```python
from build123d import *

# Parameters (mm, degrees)
EXTRUDE_2_DEPTH = 350
FILLET_1_R      = 1.5


with BuildPart() as part:
    # 草图1 → 凸台-拉伸2 (new body)
    with BuildSketch(Plane.XY):
        Polygon((-10, -3.15), (-10, -10), (-3.15, -10), (-3.15, -8.2), (-3.95, -8.2), (-3.95, -9.2), (-5.634314575, -9.2), (-5.634314575, -6.2), (-3.134314575, -3.7), (3.134314575, -3.7), (5.634314575, -6.2), (5.634314575, -9.2), (3.95, -9.2), (3.95, -8.2), (3.15, -8.2), (3.15, -10), (10, -10), (10, -3.15), (8.2, -3.15), (8.2, -3.95), (9.2, -3.95), (9.2, -5.634314575), (6.2, -5.634314575), (3.7, -3.134314575), (3.7, 3.134314575), (6.2, 5.634314575), (9.2, 5.634314575), (9.2, 3.95), (8.2, 3.95), (8.2, 3.15), (10, 3.15), (10, 10), (3.15, 10), (3.15, 8.2), (3.95, 8.2), (3.95, 9.2), (5.634314575, 9.2), (5.634314575, 6.2), (3.134314575, 3.7), (-3.134314575, 3.7), (-5.634314575, 6.2), (-5.634314575, 9.2), (-3.95, 9.2), (-3.95, 8.2), (-3.15, 8.2), (-3.15, 10), (-10, 10), (-10, 3.15), (-8.2, 3.15), (-8.2, 3.95), (-9.2, 3.95), (-9.2, 5.634314575), (-6.2, 5.634314575), (-3.7, 3.134314575), (-3.7, -3.134314575), (-6.2, -5.634314575), (-9.2, -5.634314575), (-9.2, -3.95), (-8.2, -3.95), (-8.2, -3.15), align=None)
    extrude(amount=EXTRUDE_2_DEPTH)

    # 圆角1
    fillet_1_edges = [part.edges().sort_by_distance(p)[0] for p in [
        (-10, -10, 175),
        (-10, 10, 175),
        (10, 10, 175),
        (10, -10, 175),
    ]]
    fillet(fillet_1_edges, radius=FILLET_1_R)


solid = part.part
```
Verification items for the finished model (mm, model axes). A direction names the side the tool comes from. Coordinates: 2 decimals unless noted, no trailing zeros. Answer as a JSON object with one key per item and string values. Group by question number.
(1) Tool access check on faces 5 (the face through (0, -3.7, 173)), 6 (the face through (6, 10, 173)). Record the directions out of +Z, -Z, +X, -X, +Y, -Y that give a thin tool (end or side, any length) a straight path to the whole face; none if there is none.
(2) Release check for a two-part mould opening along Y. For faces 1 (the face through (3.7, 0, 173)), 2 (the face through (-3.7, 0, 173)), 3 (the face through (0, 3.7, 173)), 4 (the face through (6, -10, 173)) record: +Y half, -Y half, draft (parallel to the pull), parting line (faces both ways), or undercut.
(3) Material ranges on line 1 (Y direction, x = -8.5, z = 218); line 2 (X direction, y = -6.5, z = 67), recorded low to high.
(4) Gauge pin test, flat ends, axial feed: pin 1 (0.5 mm diameter, centred on x = 9.5, z = 178, fed in from -Y); pin 2 (1.9 mm diameter, centred on y = 1, z = 226, fed in from +X). Record the tip position at first contact, or that the pin passes through.
Reply:
{
 "1": {"face 5": "+Z, -Z, -Y", "face 6": "+Z, -Z, +X, -X, +Y"},
 "2": {"face 1": "undercut", "face 2": "undercut", "face 3": "+Y half", "face 4": "-Y half"},
 "3": {"line 1": "-10 to -5.63, -3.95 to -3.15, 3.15 to 3.95, 5.63 to 10", "line 2": "-10 to -5.63, 5.63 to 10"},
 "4": {"pin 1": "y = -9.8", "pin 2": "x = 3.7"}
}
